Verification items for this drawing (mm, ordinates from the low corner). Give positions to 0.01 mm unless a question says otherwise; leave off trailing zeros. Order: outer loops, then holes, each group sorted by start corner. A loop starts at its lowest first (then second) coordinate and runs counter-clockwise, first axis right, second up. Notation, with made-up numbers: M 11.5,15.25 L 57.5,15.25 A24 ccw 57.5,33.25 Z; hole C 73,-15.5 d10. An arc over 180 degrees is marked long. Answer as a JSON object with one key per item and string values.
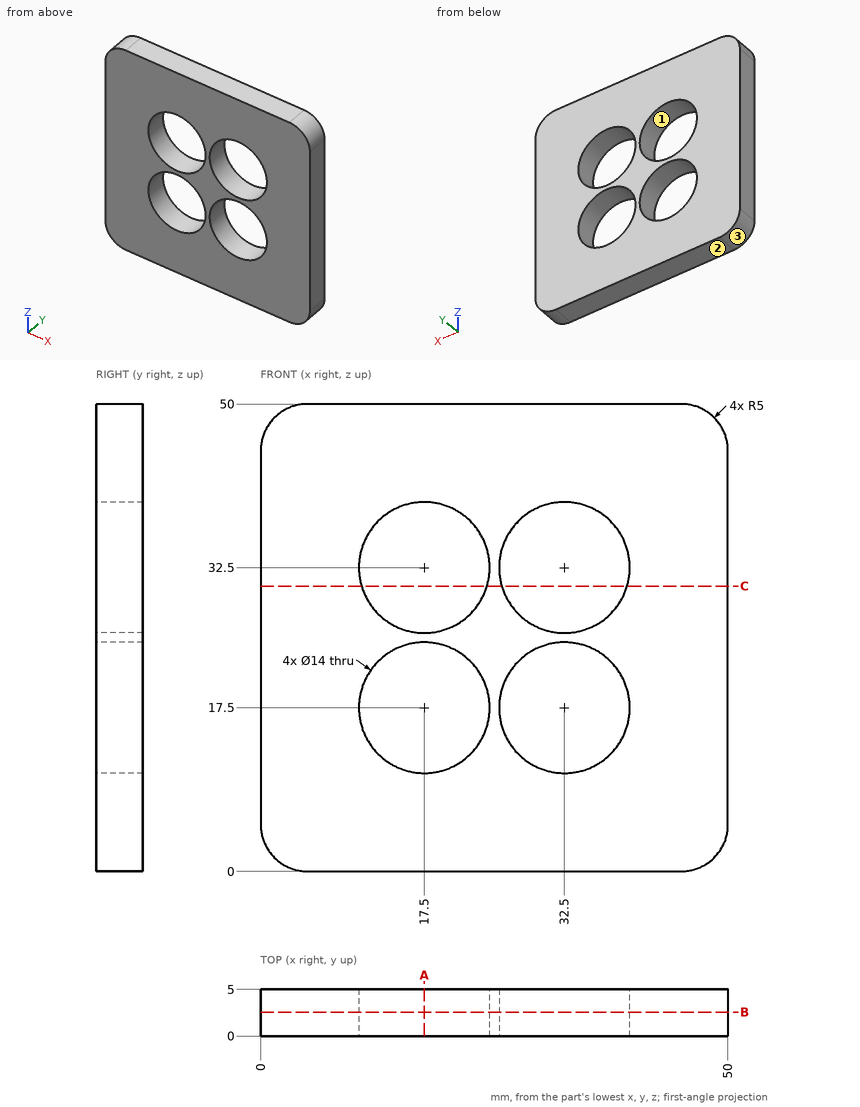
Q1. Material ranges on L1, parallel to Z at x = 17.5, y = 2.3; L2, parallel to X at y = 4.7, z = 29; L3, parallel to X at y = 4.3, z = 27.5, recorded low to high.
Resolved:
{"L1": "z = 0 to 10.5, 24.5 to 25.5, 39.5 to 50", "L2": "x = 0 to 11.44, 23.56 to 26.44, 38.56 to 50", "L3": "x = 0 to 12.6, 22.4 to 27.6, 37.4 to 50"}
Q2. Gauge pin test, flat end, axial feed: pin 1 Ø22.5 at (x, z) = (17.5, 32.5) entering from -Y. Record the tip position at first contact, or that the pin passes through.
Resolved:
{"pin 1": "stops at y = 0"}
Q3. Release check for a two-part mould opening along X. For the marked faces 1, 2 and 3 record: +X half, -X half, draft (parallel to the pull), parting line (faces both ways), or undercut.
Resolved:
{"face 1": "undercut", "face 2": "draft", "face 3": "-X half"}
Q4. Section check A-A on x = 17.5. Record the cut outline in (y, z).
Resolved:
{"outline": "M 0,0 L 5,0 L 5,10.5 L 0,10.5 Z; M 0,24.5 L 5,24.5 L 5,25.5 L 0,25.5 Z; M 0,39.5 L 5,39.5 L 5,50 L 0,50 Z"}
Q5. Section check C-C on z = 30.5. Record the cut outline in (x, y).
Resolved:
{"outline": "M 0,0 L 10.79,0 L 10.79,5 L 0,5 Z; M 24.21,0 L 25.79,0 L 25.79,5 L 24.21,5 Z; M 39.21,0 L 50,0 L 50,5 L 39.21,5 Z"}
Q6. Section check B-B on y = 2.55. Record the cut outline in (x, z), then the cut area to 3 significant figures.
Resolved:
{"outline": "M 0,5 A5 ccw 5,0 L 45,0 A5 ccw 50,5 L 50,45 A5 ccw 45,50 L 5,50 A5 ccw 0,45 Z; hole C 17.5,17.5 d14; hole C 17.5,32.5 d14; hole C 32.5,17.5 d14; hole C 32.5,32.5 d14", "area": "1,860 mm²"}
